```python
from build123d import *

# Parameters (mm, degrees)
F0_R     = 51.457531
F0_R_2   = 34.242605
F1_DEPTH = 96.266
F2_R     = 75.207579
F2_R_2   = 43.853945
F3_DEPTH = 35.052


with BuildPart() as f1:
    # F0 (on Top) → F1 (new body)
    with BuildSketch(Plane.XY):
        with Locations((0, -2.172645)):
            Circle(F0_R)
        Circle(F0_R_2, mode=Mode.SUBTRACT)
    extrude(amount=-F1_DEPTH)

    # F2 (on face) → F3 (join)
    with BuildSketch(Plane(origin=(0, 0, -96.266), x_dir=(1, 0, 0), z_dir=(0, 0, -1))):
        with Locations((1.889259, 1.605868)):
            Circle(F2_R)
        with Locations((1.889259, 1.605868)):
            Circle(F2_R_2, mode=Mode.SUBTRACT)
    extrude(amount=F3_DEPTH)


solid = f1.part
```
Geometry check sheet. Reference: the model listing, model coordinates, mm. A direction names the side the tool comes from. Round coordinates to 2 decimals unless told otherwise and drop trailing zeros. Loops run counter-clockwise (first coordinate to the right, second up) from the corner with the lowest first, then second, coordinate; pieces in that order, holes last. Notation, with made-up numbers: (-28.5, 0.5) - (-0.5, 0.5) arc R21 ccw to (-0.5, 15.5) - close; hole circle Ø2 at (49, -29.5). An arc over 180 degrees is marked (long way). Write item = value, one per line. Start each with the question number.
1. Thickness scan on line 1 (Y direction, x = 0, z = -71); line 2 (Y direction, x = 2, z = -114.5); line 3 (Z direction, x = -20, y = 67). Record the ranges inside material, lowest first.
2. Mould release check, pull along X, two halves, no side actions. Record for faces 1 (the face through (32.66, 10.29, -47.46)), 2 (the face through (18, 47, -96.266)), 3 (the face through (-40.835, -33.484, -47.459)): released by +X, released by -X, zero draft, split by the parting line, or undercut.
3. Depth check by flat-ended pin: pin 1 (10 mm diameter, centred on y = 32, z = -116, fed in from -X); pin 2 (1 mm diameter, centred on y = -48.5, z = -64.5, fed in from -X); pin 3 (3 mm diameter, centred on x = 50.5, y = 22.5, fed in from +Z). Enter the tip coordinate at first touch or a pass-through.
4. Section check D-D on z = -82. Enter the section's corners in (x, y), then the cut area to 3 significant figures.
5. Section check C-C on x = -49. Enter the section's corners in (y, z), then the cut area to 3 significant figures.
6. Section check A-A on x = 25. Enter the section's corners in (y, z).
7. Set-up check for faces 4 (the face through (43.718, -14.778, -113.547)), 5 (the face through (73.624, -24.196, -113.547)): record each of +Z, -Z, +X, -X, +Y, -Y from which the full face is reachable in a straight line by a thin tool's end or side.
8. Section check B-B on y = 32. Enter the section's corners in (x, z).
Working result:
q1.line_1 = -53.63 to -34.24, 34.24 to 49.28
q1.line_2 = -76.81 to -45.46, 42.25 to 73.6
q1.line_3 = -131.32 to -96.27
q2.face_1 = undercut
q2.face_2 = zero draft
q2.face_3 = split by the parting line
q3.pin_1 = -67.67
q3.pin_2 = -23.4
q3.pin_3 = -96.27
q4.outline = circle Ø102.92 at (0, -2.17); hole circle Ø68.49 at (0, 0)
q4.area = 4,630 mm^2
q5.outline = (-56.98, -131.32) - (53.77, -131.32) - (53.77, -96.27) - (13.54, -96.27) - (13.54, 0) - (-17.88, 0) - (-17.88, -96.27) - (-56.98, -96.27) - close
q5.area = 6,910 mm^2
q6.outline = (-73.17, -131.32) - (-38.88, -131.32) - (-38.88, -96.27) - (-23.4, -96.27) - (-23.4, 0) - (-47.15, 0) - (-47.15, -96.27) - (-73.17, -96.27) - close; (23.4, -96.27) - (35.66, -96.27) - (35.66, -131.32) - (69.96, -131.32) - (69.96, -96.27) - (42.8, -96.27) - (42.8, 0) - (23.4, 0) - close
q7.face_4 = -Z
q7.face_5 = +Z, -Z
q8.outline = (-65.39, -131.32) - (-26.29, -131.32) - (-26.29, -96.27) - (-12.19, -96.27) - (-12.19, 0) - (-38.47, 0) - (-38.47, -96.27) - (-65.39, -96.27) - close; (12.19, -96.27) - (30.06, -96.27) - (30.06, -131.32) - (69.17, -131.32) - (69.17, -96.27) - (38.47, -96.27) - (38.47, 0) - (12.19, 0) - close
